from build123d import *

# Parameters (mm, degrees)
F0_R     = 1.5
F1_DEPTH = 1.25
F2_R     = 1.24999
F3_R     = 0.5


# Not quite as in the source:
# - a fillet or chamfer is up to 0.001 mm smaller than in the source, because OpenCascade refuses the exact size


with BuildPart() as f1:
    # F0 (on Front) → F1 (new body, symmetric)
    with BuildSketch(Plane.XZ):
        with BuildLine():
            ThreePointArc((2, 16.1264534229), (0, -16.25), (-2, 16.1264534229))
            Line((-2, 16.1264534229), (-2, 24.1264534229))
            ThreePointArc((-2, 24.1264534229), (-4.1221023219, 23.2646436342), (-5.9979579511, 21.9504138084))
            Line((-5.9979579511, 21.9504138084), (-14.1837464065, 14.7155008072))
            ThreePointArc((-14.1837464065, 14.7155008072), (-20.0302422156, -8.9154770598), (0, -22.75))
            ThreePointArc((0, -22.75), (20.0302422156, -8.9154770598), (14.1837464065, 14.7155008072))
            Line((14.1837464065, 14.7155008072), (5.9979579511, 21.9504138084))
            ThreePointArc((5.9979579511, 21.9504138084), (4.1221023219, 23.2646436342), (2, 24.1264534229))
            Line((2, 24.1264534229), (2, 16.1264534229))
        make_face()
        with Locations((-5, 19.4933966718)):
            Circle(F0_R, mode=Mode.SUBTRACT)
        with Locations((5, 19.4933966718)):
            Circle(F0_R, mode=Mode.SUBTRACT)
    extrude(amount=F1_DEPTH, both=True)

    # F2 (radius 1.25 in the source; OpenCascade refuses exactly that, so slightly less here)
    f2_edges = [f1.edges().sort_by_distance(p)[0] for p in [
        (0, -1.25, -16.25),
        (0, 1.25, -16.25),
    ]]
    fillet(f2_edges, radius=F2_R)

    # F3
    f3_edges = [f1.edges().sort_by_distance(p)[0] for p in [
        (-20.030242, -1.25, -8.915477),
        (20.030242, -1.25, -8.915477),
        (-20.030242, 1.25, -8.915477),
        (20.030242, 1.25, -8.915477),
        (10.090852, 1.25, 18.332957),
        (10.090852, -1.25, 18.332957),
        (4.122102, -1.25, 23.264644),
        (4.122102, 1.25, 23.264644),
        (2, 0.625, 24.126453),
        (2, -0.625, 24.126453),
        (-10.090852, -1.25, 18.332957),
        (-10.090852, 1.25, 18.332957),
        (-4.122102, -1.25, 23.264644),
        (-4.122102, 1.25, 23.264644),
        (-2, 0.625, 24.126453),
        (-2, -0.625, 24.126453),
    ]]
    fillet(f3_edges, radius=F3_R)


solid = f1.part
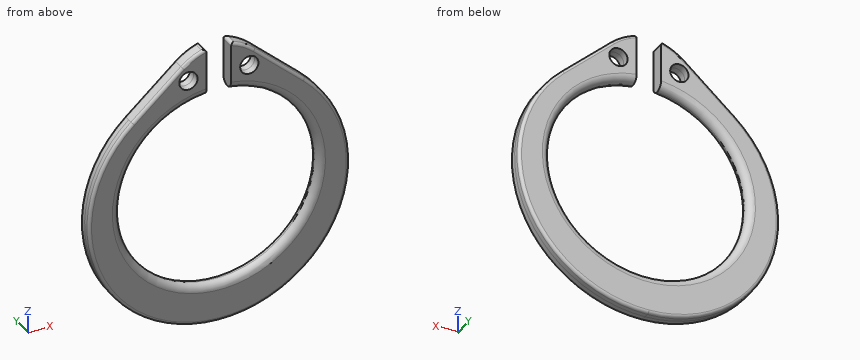
CAD build for the part. Positions are in the model's coordinates, mm. Coordinates: 2 decimals unless noted, no trailing zeros. Use one line per item in the form item = value. Start each with the question number.
1) Band-saw the part on A-A (x = 5). State how many separate pieces and enclosed holes the cut face has, and give its area (3 significant figures).
2) Flat gauge pins, fed straight in: pin 1 (2.5 mm diameter, centred on x = 5, z = 19.49, fed in from +Y); pin 2 (1 mm diameter, centred on y = -1, z = -5.5, fed in from +X); pin 3 (1 mm diameter, centred on y = 0.5, z = 2, fed in from +X); pin 4 (4 mm diameter, centred on x = -5, z = 19.49, fed in from -Y). Where does each tip first touch, or does it go through?
3) Drill centre lines: L1, parallel to Z at x = -5, y = -0.85; L2, parallel to Z at x = 5, y = -0.75; L3, parallel to X at y = 0.55, z = 0. Where is each one in solid material? Low to high. Write a range as from..to.
Check values:
q1.separate_pieces = 3
q1.enclosed_holes = 0
q1.area = 25.8 mm2
q2.pin_1 = through
q2.pin_2 = 21.09
q2.pin_3 = 21.23
q2.pin_4 = -1.25
q3.L1 = -22.15..-15.81, 15.81..17.99, 20.99..22.72
q3.L2 = -22.16..-15.72, 15.72..17.99, 20.99..22.73
q3.L3 = -21.38..-16.38, 16.38..21.38
